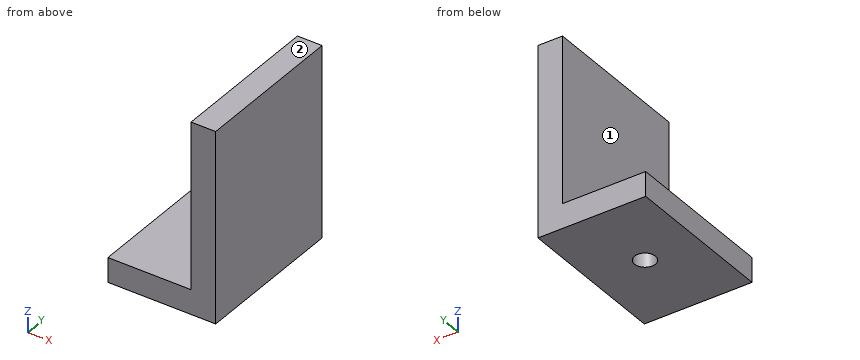
```python
from build123d import *

# Parameters (mm, degrees)
F0_W     = 27
F0_H     = 8
F1_DEPTH = 50
F3_D     = 6.8


with BuildPart() as f1:
    # F0 (on Front) → F1 (new body)
    with BuildSketch(Plane.XZ):
        with Locations((5.6900825575, -2.8987607956)):
            Rectangle(F0_W, F0_H)
        Polygon((19.1900825575, 55.1012392044), (19.1900825575, 1.1012392044), (19.1900825575, -6.8987607956), (27.1900825575, -6.8987607956), (27.1900825575, 55.1012392044), align=None)
    extrude(amount=F1_DEPTH)

    # F3 (through all)
    with Locations(Plane(origin=(0, 0, -6.8987607956), x_dir=(1, 0, 0), z_dir=(0, 0, -1))):
        with Locations((9.6900825575, 25)):
            Hole(F3_D / 2)


solid = f1.part
```
Build history of the part. All positions in model axes, mm. Face numbers are marked on the shaded views. A direction names the side the tool comes from. Coordinates: 2 decimals unless noted, no trailing zeros. Write each loop counter-clockwise with the first axis right and the second up, starting at its lowest first coordinate (ties: lowest second). Pieces come first, ordered by that corner, then holes.
1. Drill centre lines: probe 1 along X at (y, z) = (-25, -4); probe 2 along X at (y, z) = (-29, 25); probe 3 along Z at (x, y) = (15, -27). Where is each one in solid material? Low to high.
Answer block:
probe 1: x = -7.81 to 6.29, 13.09 to 27.19
probe 2: x = 19.19 to 27.19
probe 3: z = -6.9 to 1.1
2. Drop flat-ended pins along their axis: pin 1 (6 mm diameter, centred on x = 6.5, z = 3, fed in from -Y); pin 2 (10 mm diameter, centred on y = -33.5, z = 11.5, fed in from -X); pin 3 (2 mm diameter, centred on x = 15.5, y = -40, fed in from +Z); pin 4 (1.5 mm diameter, centred on x = 16.5, z = 25, fed in from -Y). Give the stop position or say it passes through.
Answer block:
pin 1: stops at y = -50
pin 2: stops at x = 19.19
pin 3: stops at z = 1.1
pin 4: passes through
3. Band-saw the part on B-B, the plane z = -2. Give the cut face in (x, y).
Answer block:
outline: (-7.81, -50) - (27.19, -50) - (27.19, 0) - (-7.81, 0) - close; hole circle Ø6.8 at (9.69, -25)
4. Band-saw the part on A-A, the plane y = -25. Give the cut face in (x, z), and give its area (3 significant figures).
Answer block:
outline: (-7.81, -6.9) - (6.29, -6.9) - (6.29, 1.1) - (-7.81, 1.1) - close; (13.09, -6.9) - (27.19, -6.9) - (27.19, 55.1) - (19.19, 55.1) - (19.19, 1.1) - (13.09, 1.1) - close
area: 658 mm2
5. Band-saw the part on D-D, the plane y = -7.5. Give the cut face in (x, z).
Answer block:
outline: (-7.81, -6.9) - (27.19, -6.9) - (27.19, 55.1) - (19.19, 55.1) - (19.19, 1.1) - (-7.81, 1.1) - close
6. Band-saw the part on C-C, the plane x = 0.5. Give the cut face in (y, z).
Answer block:
outline: (-50, -6.9) - (0, -6.9) - (0, 1.1) - (-50, 1.1) - close
7. 3-axis set-ups, long thin cutter, end or side, ignore diameter. For the marked faces 1 and 2: which of +Z, -Z, +X, -X, +Y, -Y reach the whole face in a straight line?
Answer block:
face 1: +Z, -X, +Y, -Y
face 2: +Z, +X, -X, +Y, -Y
